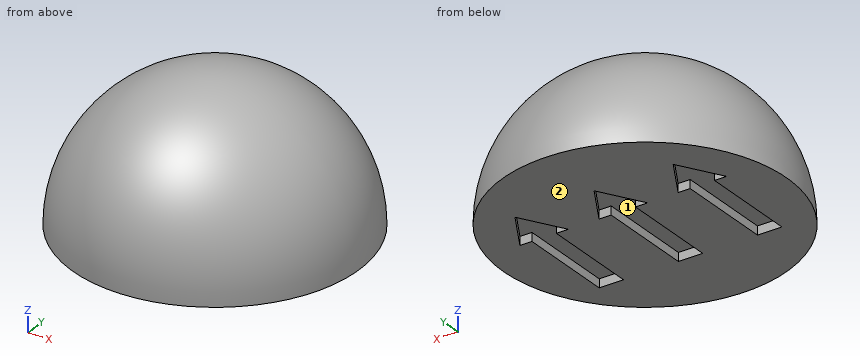
```python
from build123d import *

# Parameters (mm, degrees)
EXTRUDE002_DEPTH = 3
EXTRUDE003_DEPTH = 3
EXTRUDE001_DEPTH = 3
RECTANGLE_W      = 100
RECTANGLE_H      = 100
EXTRUDE_DEPTH    = 50


with BuildPart() as extrude002:
    # Fusion001 → Extrude002 (new body)
    with BuildSketch(Plane(origin=(-45, 30, 0), x_dir=(1, 0, 0), z_dir=(0, 0, 1))):
        Polygon((17.44346, -4.685924), (26.023636, -19.546554), (21.745595, -19.546554), (21.745595, -53.769589), (13.140465, -53.769589), (13.140465, -19.546554), (8.861994, -19.546554), align=None)
    extrude(amount=EXTRUDE002_DEPTH)


with BuildPart() as extrude003:
    # Fusion002 → Extrude003 (new body)
    with BuildSketch(Plane(origin=(11, 30, 0), x_dir=(1, 0, 0), z_dir=(0, 0, 1))):
        Polygon((17.44346, -4.685924), (26.023636, -19.546554), (21.745595, -19.546554), (21.745595, -53.769589), (13.140465, -53.769589), (13.140465, -19.546554), (8.861994, -19.546554), align=None)
    extrude(amount=EXTRUDE003_DEPTH)


with BuildPart() as extrude001:
    # Fusion → Extrude001 (new body)
    with BuildSketch(Plane(origin=(-17, 30, 0), x_dir=(1, 0, 0), z_dir=(0, 0, 1))):
        Polygon((17.44346, -4.685924), (26.023636, -19.546554), (21.745595, -19.546554), (21.745595, -53.769589), (13.140465, -53.769589), (13.140465, -19.546554), (8.861994, -19.546554), align=None)
    extrude(amount=EXTRUDE001_DEPTH)


with BuildPart() as extrude_body:
    # Rectangle → Extrude (new body)
    with BuildSketch(Plane(origin=(-50, 50, 0), x_dir=(1, 0, 0), z_dir=(0, 0, 1))):
        with Locations((50, -50)):
            Rectangle(RECTANGLE_W, RECTANGLE_H)
    extrude(amount=-EXTRUDE_DEPTH)


with BuildPart() as obj1:
    # Sphere → Sphere (revolve)
    with BuildSketch(Plane.XZ):
        with BuildLine():
            ThreePointArc((0, -50), (50, 0), (0, 50))
            Line((0, 50), (0, -50))
        make_face()
    revolve(axis=Axis((0, 0, 0), (0, 0, 1)))

    # Cut: cut Extrude body
    add(extrude_body.part, mode=Mode.SUBTRACT)

    # Cut002: cut Extrude001
    add(extrude001.part, mode=Mode.SUBTRACT)

    # Cut003: cut Extrude003
    add(extrude003.part, mode=Mode.SUBTRACT)

    # Cut004: cut Extrude002
    add(extrude002.part, mode=Mode.SUBTRACT)


solid = obj1.part
```
Geometry check sheet. Reference: the model listing, model coordinates, mm. Face numbers are marked on the shaded views. Round coordinates to 2 decimals unless told otherwise and drop trailing zeros. Loops run counter-clockwise (first coordinate to the right, second up) from the corner with the lowest first, then second, coordinate; pieces in that order, holes last. Notation, with made-up numbers: (34, 9.25) - (66, 9.25) arc R22 cw to (66, 38.25) - close; hole circle Ø2 at (-13, -35). An arc over 180 degrees is marked (long way). Write each question's results on one line, items separated by ' | '. Start each with the question number.
Q1. Cross-section at A-A on y = -22.5. Enter the section's corners in (x, z), and give its area (3 significant figures).
Q2. Thickness scan on line 1 (Z direction, x = -43, y = -3); line 2 (Z direction, x = -4.5, y = -37); line 3 (Y direction, x = -23.5, z = 19). Record the ranges inside material, lowest first. Write a range as [from, to].
Q3. Gauge pin test, flat ends, axial feed: P1, Ø5, axis at x = 25, z = 9, coming from the +Y side; P2, Ø0.9, axis at x = -20.5, z = 1, coming from the +Y side; P3, Ø5, axis at y = 17, z = 14, coming from the +X side. Record the tip position at first contact, or that the pin passes through.
Q4. Cross-section at D-D on y = -5. Enter the section's corners in (x, z).
Q5. Release check for a two-part mould opening along Y. For the marked faces 1 and 2 record: +Y half, -Y half, draft (parallel to the pull), parting line (faces both ways), or undercut.
Q6. Cross-section at C-C on x = -26. Enter the section's corners in (y, z), and give its area (3 significant figures).
Q7. Cross-section at B-B on z = 14. Enter the section's corners in (x, y), and give its area (3 significant figures).
Answers below:
1) outline: (-44.65, 0) - (-31.86, 0) - (-31.86, 3) - (-23.25, 3) - (-23.25, 0) - (-3.86, 0) - (-3.86, 3) - (4.75, 3) - (4.75, 0) - (24.14, 0) - (24.14, 3) - (32.75, 3) - (32.75, 0) - (44.65, 0) arc R44.65 ccw to start | area: 3,050 mm²
2) line 1: z = [0, 25.34] | line 2: z = [0, 33.33] | line 3: y = [-39.83, 39.83]
3) P1: stops at y = 43.82 | P2: stops at y = 45.79 | P3: stops at x = 46.03
4) outline: (-49.75, 0) - (-31.86, 0) - (-31.86, 3) - (-23.25, 3) - (-23.25, 0) - (-3.86, 0) - (-3.86, 3) - (4.75, 3) - (4.75, 0) - (24.14, 0) - (24.14, 3) - (32.75, 3) - (32.75, 0) - (49.75, 0) arc R49.75 ccw to start
5) face 1: undercut | face 2: draft
6) outline: (-42.71, 0) - (-23.77, 0) - (-23.77, 3) - (22.62, 3) - (22.62, 0) - (42.71, 0) arc R42.71 ccw to start | area: 2,730 mm²
7) outline: circle Ø96 at (0, 0) | area: 7,240 mm²
